Source: CAD feature listing. Evaluate the final solid. Frame: model axes, mm. A direction names the side the tool comes from. Coordinates: 2 decimals unless noted, no trailing zeros. Write each loop counter-clockwise with the first axis right and the second up, starting at its lowest first coordinate (ties: lowest second). Pieces come first, ordered by that corner, then holes. Notation, with made-up numbers: (-17, -29.75) -> (39, -29.75) arc R16 cw to (39, -4.75) -> close; hole circle Ø10 at (-38, 78.25). An arc over 180 degrees is marked (long way). One line per item, written item: value. Start each with the question number.
1. Access query for faces 1 (the cylindrical face through (-7.4, 3.1, 2.8)), 2 (the flat face through (103, 7, 17)). Directions: +Z, -Z, +X, -X, +Y, -Y. A direction counts if a zero-diameter tool reaches every point of the face in a straight line with its end or side. Return the directions, or none.
2. Section query C-C, the plane z = 2. Output: boundary loops of the cut face in (x, y).
3. First-contact query: P1, Ø1.5, axis at y = 12, z = 22, coming from the -X side. Flat tip, straight axial feed; report the tip coordinate or a pass-through.
4. Section query A-A, the plane x = -2.5. Output: boundary loops of the cut face in (y, z), and give its area (3 significant figures).
5. Section query D-D, the plane y = 11. Output: boundary loops of the cut face in (x, z), and give its area (3 significant figures).
6. Section query B-B, the plane y = 2.5. Output: boundary loops of the cut face in (x, z).
7. Line query: line 1 (X direction, y = 7.5, z = 3). Output: solid intervals per line, ascending.
from build123d import *

# Parameters (mm, degrees)
SKETCH1_W           = 103
SKETCH1_H           = 15
BOSS_EXTRUDE1_DEPTH = 34
SKETCH2_R           = 1
BOSS_EXTRUDE2_DEPTH = 15


with BuildPart() as part:
    # Sketch1 → Boss-Extrude1 (new body)
    with BuildSketch(Plane.XY):
        with Locations((51.5, 7.5)):
            Rectangle(SKETCH1_W, SKETCH1_H)
    extrude(amount=BOSS_EXTRUDE1_DEPTH)

    # Sketch2 → Boss-Extrude2 (add)
    with BuildSketch(Plane.ZY):
        with Locations(Location((2, 2.5, 0), (0, 0, 180))):
            Circle(SKETCH2_R)
        with Locations(Location((2, 4.6, 0), (0, 0, 180))):
            Circle(SKETCH2_R)
    extrude(amount=BOSS_EXTRUDE2_DEPTH)


solid = part.part
Computed values:
1. face 1: -X
1. face 2: +Z, -Z, +X, +Y, -Y
2. outline: (-15, 1.5) -> (0, 1.5) -> (0, 0) -> (103, 0) -> (103, 15) -> (0, 15) -> (0, 5.6) -> (-15, 5.6) -> (-15, 3.6) -> (0, 3.6) -> (0, 3.5) -> (-15, 3.5) -> close
3. P1: stops at x = 0
4. outline: circle Ø2 at (2.5, 2); circle Ø2 at (4.6, 2)
4. area: 6.28 mm²
5. outline: (0, 0) -> (103, 0) -> (103, 34) -> (0, 34) -> close
5. area: 3,500 mm²
6. outline: (-15, 1) -> (0, 1) -> (0, 0) -> (103, 0) -> (103, 34) -> (0, 34) -> (0, 3) -> (-15, 3) -> close
7. line 1: x = 0 to 103
